For this review, take the finished solid that the model builds, in its own axes (mm). A direction names the side the tool comes from. Give positions to 0.01 mm unless a question says otherwise; leave off trailing zeros. Loops run counter-clockwise (first coordinate to the right, second up) from the corner with the lowest first, then second, coordinate; pieces in that order, holes last. Notation, with made-up numbers: M 1.25,44 L 55.25,44 A17 ccw 55.25,75 Z; hole C 1.5,38.25 d5. An arc over 180 degrees is marked long. Use CSV: the item, a comma, the result in double quotes. Start each with the question number.
1. Take a section at C-C, the plane z = 8.25. Write out the cut boundary in (x, y), and give its area (3 significant figures).
2. Tool access review of faces 1 (the face through (3.6, 1, 0)), 2 (the face through (2, 1.8, -1)), 3 (the face through (4.25, -2, 7)): name each direction out of +Z, -Z, +X, -X, +Y, -Y from which nothing blocks a thin tool from reaching the whole face with its end or side.
3. Take a section at B-B, the plane z = -0.5. State how many separate pieces and enclosed holes the cut face has, and give its area (3 significant figures).
4. Take a section at D-D, the plane x = 1. Write out the cut boundary in (y, z).
5. Take a section at A-A, the plane y = 0.5. Write out the cut boundary in (x, z).
6. The part is to be moulded in two halves that separate along X. For faces 4 (the face through (-3.268, 3.969, -0.836)), 5 (the face through (0, 1, 2)), 6 (the face through (-4.25, -2, 7)), 7 (the face through (0, 1.8, -2)), say which applies: pulls with the +X half, pulls with the -X half, needs draft (parallel to the pull), parting line crosses it, or undercut.
7. To check wall thickness, follow line 1 (X direction, y = 0.6, z = 0); line 2 (Y direction, x = -1.5, z = 6); line 3 (Y direction, x = 0.75, z = 3.5). State the ranges of each line that lie inside material, in increasing order. Write a range as [from, to].
8. Insertion check: P1, Ø6, axis at x = 4, z = 1.5, coming from the -Y side; P2, Ø2, axis at x = 2, z = 6.5, coming from the +Y side; P3, Ø1.9, axis at x = 1.755, z = -0.5, coming from the +Y side. Each pin has a flat end and moves straight along its axis. Give the tip position at first contact, or say it passes through.
from build123d import *

# Parameters (mm, degrees)
SKETCH_2_R          = 0.9
EXTRUDE_1_DEPTH     = 0.8
SKETCH_3_W          = 7.2
SKETCH_3_H          = 5
EXTRUDE_2_DEPTH     = 1
SKETCH_4_R          = 1.75
SKETCH_4_R_2        = 1.55
EXTRUDE_5_DEPTH     = 4.4
SKETCH_6_W          = 8.5
SKETCH_6_H          = 4
EXTRUDE_6_DEPTH     = 4.1
SKETCH_7_W          = 8.1
SKETCH_7_H          = 3.7
CUT_EXTRUDE_1_DEPTH = 3.8


with BuildPart() as part:
    # 草图2 → 凸台-拉伸1 (new body)
    with BuildSketch(Plane(origin=(0, 0, 0), x_dir=(1, 0, 0), z_dir=(0, 1, 0))):
        with BuildLine():
            Line((-6.5, 3), (6.5, 3))
            ThreePointArc((6.5, 3), (9.5, 0), (6.5, -3))
            Line((6.5, -3), (5, -3))
            Line((5, -3), (5, -9))
            Line((5, -9), (-5, -9))
            Line((-5, -9), (-5, -3))
            Line((-5, -3), (-6.5, -3))
            ThreePointArc((-6.5, -3), (-9.5, 0), (-6.5, 3))
        make_face()
        with Locations(Location((-6.5, 0, 0), (0, 0, 270))):
            Circle(SKETCH_2_R, mode=Mode.SUBTRACT)
        with Locations(Location((6.5, 0, 0), (0, 0, 270))):
            Circle(SKETCH_2_R, mode=Mode.SUBTRACT)
    extrude(amount=EXTRUDE_1_DEPTH)

    # 草图3 → 凸台-拉伸2 (add)
    with BuildSketch(Plane(origin=(0, 0.8, 0), x_dir=(1, 0, 0), z_dir=(0, 1, 0))):
        with Locations((0, 0.5)):
            Rectangle(SKETCH_3_W, SKETCH_3_H)
    extrude(amount=EXTRUDE_2_DEPTH)

    # 草图4 → 凸台-拉伸5 (add)
    # profile 1 of 2: a face of its own
    with BuildSketch(Plane(origin=(0, 1.8, 0), x_dir=(1, 0, 0), z_dir=(0, 1, 0))):
        with Locations(Location((-1.755, 0.5, 0), (0, 0, 270))):
            Circle(SKETCH_4_R)
        with Locations(Location((-1.755, 0.5, 0), (0, 0, 270))):
            Circle(SKETCH_4_R_2, mode=Mode.SUBTRACT)
    # profile 2 of 2: a face of its own
    with BuildSketch(Plane(origin=(0, 1.8, 0), x_dir=(1, 0, 0), z_dir=(0, 1, 0))):
        with Locations(Location((1.755, 0.5, 0), (0, 0, 90))):
            Circle(SKETCH_4_R)
        with Locations(Location((1.755, 0.5, 0), (0, 0, 90))):
            Circle(SKETCH_4_R_2, mode=Mode.SUBTRACT)
    extrude(amount=EXTRUDE_5_DEPTH)

    # 草图6 → 凸台-拉伸6 (add)
    with BuildSketch(Plane.XZ):
        with Locations((0, 7)):
            Rectangle(SKETCH_6_W, SKETCH_6_H)
    extrude(amount=EXTRUDE_6_DEPTH)

    # 草图7 → 切除-拉伸1 (cut)
    with BuildSketch(Plane.XY.offset(9)):
        with Locations((0, -2.05)):
            Rectangle(SKETCH_7_W, SKETCH_7_H)
    extrude(amount=-CUT_EXTRUDE_1_DEPTH, mode=Mode.SUBTRACT)


solid = part.part
Result set:
1,outline,"M -5,0 L -4.25,0 L -4.25,-4.1 L 4.25,-4.1 L 4.25,0 L 5,0 L 5,0.8 L -5,0.8 Z; hole M -4.05,-3.9 L 4.05,-3.9 L 4.05,-0.2 L -4.05,-0.2 Z"
1,area,"12.9 mm2"
2,face 1,"+Z, -Z, +X, +Y"
2,face 2,"+Y"
2,face 3,"+Z, -Z, +X, -Y"
3,separate pieces,"3"
3,enclosed holes,"0"
3,area,"23.5 mm2"
4,outline,"M -4.1,5 L 0,5 L 0,-3 L 1.8,-3 L 1.8,-2.08 L 6.2,-2.08 L 6.2,-1.85 L 1.8,-1.85 L 1.8,0.85 L 6.2,0.85 L 6.2,1.08 L 1.8,1.08 L 1.8,2 L 0.8,2 L 0.8,9 L -0.2,9 L -0.2,5.2 L -3.9,5.2 L -3.9,9 L -4.1,9 Z"
5,outline,"M -6.5,-3 L 6.5,-3 A3 ccw 6.5,3 L 5,3 L 5,9 L -5,9 L -5,3 L -6.5,3 A3 ccw Z; hole C -6.5,0 d1.8; hole C 6.5,0 d1.8"
6,face 4,"undercut"
6,face 5,"needs draft"
6,face 6,"pulls with the -X half"
6,face 7,"undercut"
7,line 1,"[-9.5, -7.4], [-5.6, 5.6], [7.4, 9.5]"
7,line 2,"[-4.1, -3.9], [-0.2, 0.8]"
7,line 3,"[0, 0.8]"
8,P1,"y = 0"
8,P2,"y = 0.8"
8,P3,"y = 1.8"
